Part print with two shaded views. Sizes in mm from the minimum x, y, z corner. Give positions to 0.01 mm unless a question says otherwise; leave off trailing zeros. Write each loop counter-clockwise with the first axis right and the second up, starting at its lowest first coordinate (ties: lowest second). Pieces come first, ordered by that corner, then holes. Notation, with made-up numbers: (9.5, -11) -> (20.5, -11) arc R21 cw to (20.5, 12) -> close; hole circle Ø1 at (-39.5, 44.25). An arc over 180 degrees is marked (long way). Write item = value, one per line. Start each with the question number.
Q1. Saw through at B-B, the plane x = 55.5. List the corners of the cut face in (y, z).
Q2. Saw through at A-A, the plane y = 10. List the corners of the cut face in (x, z).
Q3. Drop flat-ended pins along their axis: P1, Ø6.5, axis at y = 8.5, z = 15, coming from the -X side; P2, Ø6.5, axis at y = 8, z = 21.5, coming from the +X side; P3, Ø6.5, axis at x = 260.5, y = 5.5, coming from the -Z side. Give the stop position or say it passes through.
Q4. Wall check: line 1 (Z direction, x = 242.5, y = 6.25); line 2 (X direction, y = 4, z = 23). Give the ranges that are in metal, low to high.
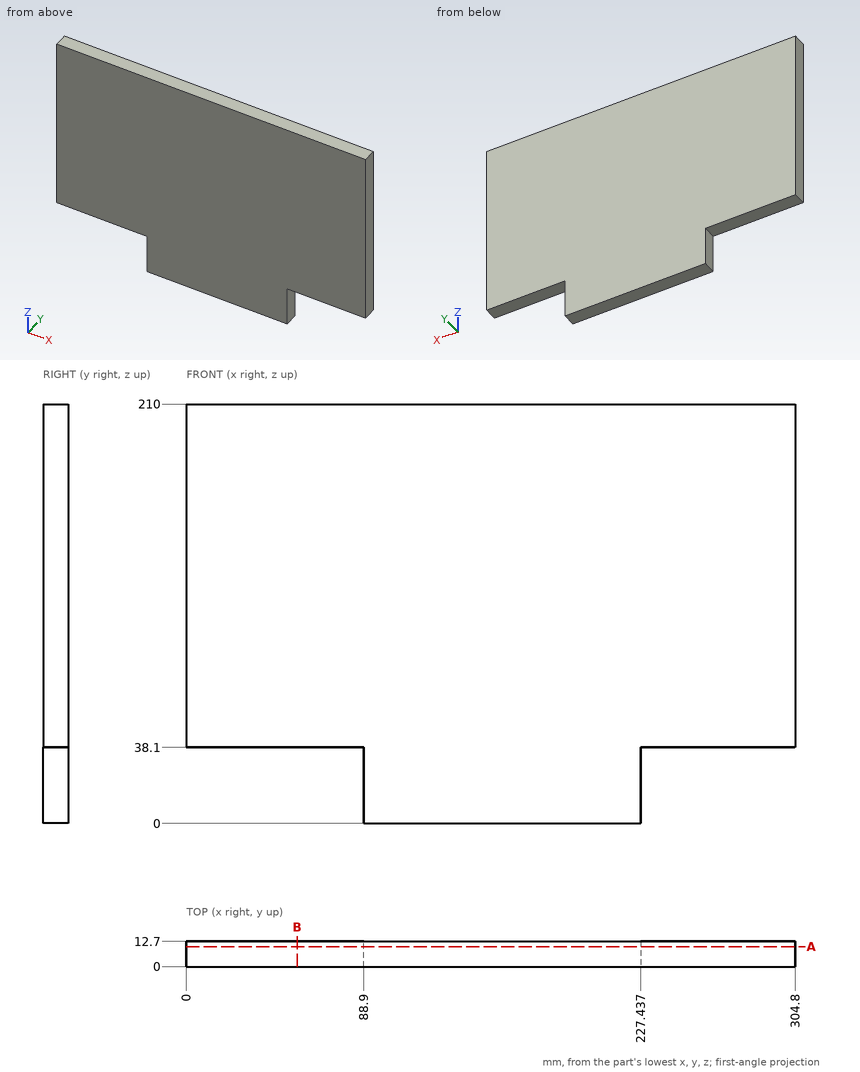
Report:
q1.outline = (0, 38.1) -> (12.7, 38.1) -> (12.7, 210) -> (0, 210) -> close
q2.outline = (0, 38.1) -> (88.9, 38.1) -> (88.9, 0) -> (227.44, 0) -> (227.44, 38.1) -> (304.8, 38.1) -> (304.8, 210) -> (0, 210) -> close
q3.P1 = 88.9
q3.P2 = 227.44
q3.P3 = 38.1
q4.line_1 = 38.1 to 210
q4.line_2 = 88.9 to 227.44
